Check sheet for the modelled part. Datum: model origin and axes. Units: mm. Face numbers are marked on the shaded views. A direction names the side the tool comes from. Give positions to 0.01 mm unless a question says otherwise; leave off trailing zeros. Order: outer loops, then holes, each group sorted by start corner. A loop starts at its lowest first (then second) coordinate and runs counter-clockwise, first axis right, second up.
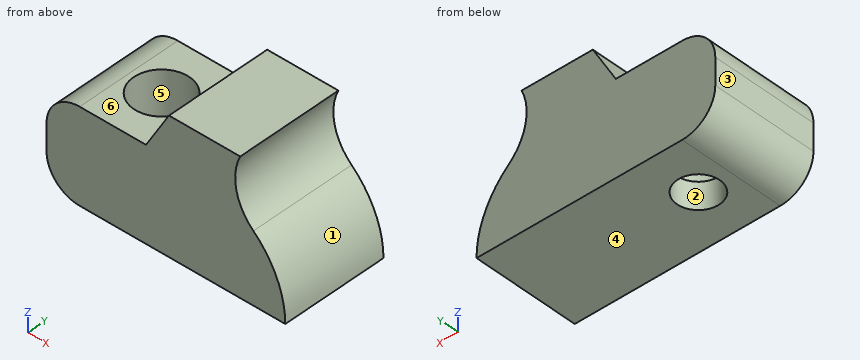
from build123d import *

# Parameters (mm, degrees)
SKETCH1_W               = 18
SKETCH1_H               = 8
SKETCH1_R               = 1.6
BOSS_EXTRUDE1_DEPTH     = 10
CUT_EXTRUDE1_DEPTH      = 1
CUT_EXTRUDE1_DEPTH_BACK = 9
CUT_EXTRUDE3_DEPTH      = 1
CUT_EXTRUDE3_DEPTH_BACK = 9
FILLET1_R               = 2.5
SKETCH4_R               = 2.1
CUT_EXTRUDE4_DEPTH      = 4
CUT_EXTRUDE4_DEPTH_BACK = 5


with BuildPart() as part:
    # Sketch1 → Boss-Extrude1 (new body)
    with BuildSketch(Plane.XY):
        with Locations((4, 0.027746394)):
            Rectangle(SKETCH1_W, SKETCH1_H)
        Circle(SKETCH1_R, mode=Mode.SUBTRACT)
    extrude(amount=BOSS_EXTRUDE1_DEPTH)

    # Sketch2 → Cut-Extrude1 (cut, two sides)
    with BuildSketch(Plane.XZ.offset(3.972253606)) as cut_extrude1_sk:
        with BuildLine():
            Line((13.221576202, 12.297519941), (13, 0))
            ThreePointArc((13, 0), (12.370590218, 2.900961957), (10.595548492, 5.280239962))
            ThreePointArc((10.595548492, 5.280239962), (9.475303393, 9.699461467), (13.221576202, 12.297519941))
        make_face()
    extrude(amount=CUT_EXTRUDE1_DEPTH, mode=Mode.SUBTRACT)
    extrude(cut_extrude1_sk.sketch, amount=-CUT_EXTRUDE1_DEPTH_BACK, mode=Mode.SUBTRACT)

    # Sketch3 → Cut-Extrude3 (cut, two sides)
    with BuildSketch(Plane(origin=(0, 4.027746394, 0), x_dir=(1, 0, 0), z_dir=(0, 1, 0))) as cut_extrude3_sk:
        Polygon((-5, -7), (2.5, -7), (4.232050808, -10), (-5, -10), align=None)
    extrude(amount=CUT_EXTRUDE3_DEPTH, mode=Mode.SUBTRACT)
    extrude(cut_extrude3_sk.sketch, amount=-CUT_EXTRUDE3_DEPTH_BACK, mode=Mode.SUBTRACT)

    # Fillet1
    fillet1_edges = [part.edges().sort_by_distance(p)[0] for p in [
        (-5, 0.027746394, 7),
        (-5, 0.027746394, 0),
    ]]
    fillet(fillet1_edges, radius=FILLET1_R)

    # Sketch4 → Cut-Extrude4 (cut, two sides)
    with BuildSketch(Plane.XY.offset(7)) as cut_extrude4_sk:
        Circle(SKETCH4_R)
    extrude(amount=CUT_EXTRUDE4_DEPTH, mode=Mode.SUBTRACT)
    extrude(cut_extrude4_sk.sketch, amount=-CUT_EXTRUDE4_DEPTH_BACK, mode=Mode.SUBTRACT)


solid = part.part
1) Set-up check for the marked faces 4, 5 and 6: record each of +Z, -Z, +X, -X, +Y, -Y from which the full face is reachable in a straight line by a thin tool's end or side.
Recorded:
face 4: -Z, +X, -X, +Y, -Y
face 5: +Z
face 6: +Z, -X, +Y, -Y
2) Section check A-A, the plane x = 0. Record the cut outline in (y, z).
Recorded:
outline: (-3.97, 0) - (-1.6, 0) - (-1.6, 2) - (-2.1, 2) - (-2.1, 7) - (-3.97, 7) - close; (1.6, 0) - (4.03, 0) - (4.03, 7) - (2.1, 7) - (2.1, 2) - (1.6, 2) - close
3) Material ranges on L1, parallel to Y at x = 0.5, z = 2.75; L2, parallel to Y at x = 0, z = 5.5; L3, parallel to X at y = 0, z = 0.4, recorded low to high.
Recorded:
L1: y = -3.97 to -2.04, 2.04 to 4.03
L2: y = -3.97 to -2.1, 2.1 to 4.03
L3: x = -3.86 to -1.6, 1.6 to 12.99
4) Draft check along X on the marked faces 1, 2 and 3. Enter one of: +X half, -X half, draft (parallel to the pull), parting line (faces both ways), or undercut.
Recorded:
face 1: +X half
face 2: undercut
face 3: -X half
5) Section check B-B, the plane y = 0. Record the cut outline in (x, z), then the cut area to 3 significant figures.
Recorded:
outline: (-5, 2.5) arc R2.5 ccw to (-2.5, 0) - (-1.6, 0) - (-1.6, 2) - (-2.1, 2) - (-2.1, 7) - (-2.5, 7) arc R2.5 ccw to (-5, 4.5) - close; (1.6, 0) - (13, 0) arc R7 ccw to (10.6, 5.28) arc R4 cw to (9.6, 10) - (4.23, 10) - (2.5, 7) - (2.1, 7) - (2.1, 2) - (1.6, 2) - close
area: 105 mm2
6) Section check D-D, the plane x = 11.75. Record the cut outline in (y, z), then the cut area to 3 significant figures.
Recorded:
outline: (-3.97, 0) - (4.03, 0) - (4.03, 3.99) - (-3.97, 3.99) - close
area: 31.9 mm2
7) Depth check by flat-ended pin: pin 1 Ø3.5 at (x, y) = (0, 0) entering from +Z; pin 2 Ø4.5 at (x, y) = (0.5, 0) entering from +Z. Enter the tip coordinate at first touch or a pass-through.
Recorded:
pin 1: stops at z = 2
pin 2: stops at z = 7.43
8) Section check C-C, the plane z = 4. Record the cut outline in (x, y).
Recorded:
outline: (-5, -3.97) - (11.74, -3.97) - (11.74, 4.03) - (-5, 4.03) - close; hole circle Ø4.2 at (0, 0)
